Here's how the part is built. I have some questions about the finished solid (model axes, mm). Face numbers are marked on the shaded views. A direction names the side the tool comes from. Round coordinates to 2 decimals unless told otherwise and drop trailing zeros. Write each loop counter-clockwise with the first axis right and the second up, starting at its lowest first coordinate (ties: lowest second). Pieces come first, ordered by that corner, then holes. Notation, with made-up numbers: (-6.75, 20) -> (52.25, 20) arc R21 ccw to (52.25, 51) -> close; hole circle Ø5 at (44.5, 78.5). An arc over 180 degrees is marked (long way). Answer as CSV lines item,"result".
```python
from build123d import *

# Parameters (mm, degrees)
SKETCH1_R               = 3.75
SKETCH1_R_2             = 2.5
BOSS_EXTRUDE1_DEPTH     = 3
SKETCH2_R               = 5
SKETCH2_R_2             = 1.25
BOSS_EXTRUDE2_DEPTH     = 20
CUT_EXTRUDE1_START      = -19
SKETCH3_R               = 3.75
CUT_EXTRUDE1_DEPTH      = 19
CHAMFER1_SIZE           = 1.5
CUT_EXTRUDE2_DEPTH      = 25.062418831
CUT_EXTRUDE2_DEPTH_BACK = 25.062418831
SKETCH4_W               = 0.5
SKETCH4_H               = 32.118567902


with BuildPart() as part:
    # Sketch1 → Boss-Extrude1 (new body)
    with BuildSketch(Plane(origin=(0, 0, 0), x_dir=(1, 0, 0), z_dir=(0, 1, 0))):
        with Locations(Location((0, 0, 0), (0, 0, 270))):
            Circle(SKETCH1_R)
        with Locations(Location((0, 0, 0), (0, 0, 270))):
            Circle(SKETCH1_R_2, mode=Mode.SUBTRACT)
    extrude(amount=BOSS_EXTRUDE1_DEPTH)

    # Sketch2 → Boss-Extrude2 (add)
    with BuildSketch(Plane(origin=(0, 3, 0), x_dir=(1, 0, 0), z_dir=(0, 1, 0))):
        with Locations(Location((0, 0, 0), (0, 0, 270))):
            Circle(SKETCH2_R)
        with Locations(Location((0, 0, 0), (0, 0, 270))):
            Circle(SKETCH2_R_2, mode=Mode.SUBTRACT)
    extrude(amount=BOSS_EXTRUDE2_DEPTH)

    # Sketch3 → Cut-Extrude1 (cut)
    with BuildSketch(Plane(origin=(0, 23, 0), x_dir=(1, 0, 0), z_dir=(0, 1, 0)).offset(CUT_EXTRUDE1_START)):
        with Locations(Location((0, 0, 0), (0, 0, 270))):
            Circle(SKETCH3_R)
    extrude(amount=CUT_EXTRUDE1_DEPTH, mode=Mode.SUBTRACT)

    # Chamfer1
    # the kernel refuses this chamfer: 1.5 mm, written as the material it adds along each edge
    with BuildSketch(Plane(origin=(0, 3, 0), x_dir=(0, 0, 1), z_dir=(-1, 0, 0))) as chamfer1_piece_1_section:
        Polygon((3.75 + CHAMFER1_SIZE, 0), (3.75, -CHAMFER1_SIZE), (3.75, 0), align=None)
    chamfer1_piece_1 = revolve(axis=Axis((0, 3, 0), (0, 1, 0)), mode=Mode.PRIVATE)
    chamfer1_piece_1 = chamfer1_piece_1 & Plane(origin=(0, 2.126111001, 0), x_dir=(0, 0, 1), z_dir=(0, -1, 0)) * Cylinder(5, 22, mode=Mode.PRIVATE)
    add(chamfer1_piece_1)
    with BuildSketch(Plane(origin=(0, 4, 0), x_dir=(0, 0, 1), z_dir=(-1, 0, 0))) as chamfer1_piece_2:
        Polygon((3.75, CHAMFER1_SIZE), (3.75 - CHAMFER1_SIZE, 0), (3.75, 0), align=None)
    revolve(axis=Axis((0, 4, 0), (0, 1, 0)))

    # Sketch4 → Cut-Extrude2 (cut, two sides: drawn at the far end of the back side and taken through both)
    with BuildSketch(Plane.XY.offset(-CUT_EXTRUDE2_DEPTH_BACK)):
        with Locations((0, 23)):
            Rectangle(SKETCH4_W, SKETCH4_H)
    extrude(amount=CUT_EXTRUDE2_DEPTH + CUT_EXTRUDE2_DEPTH_BACK, mode=Mode.SUBTRACT)


solid = part.part
```
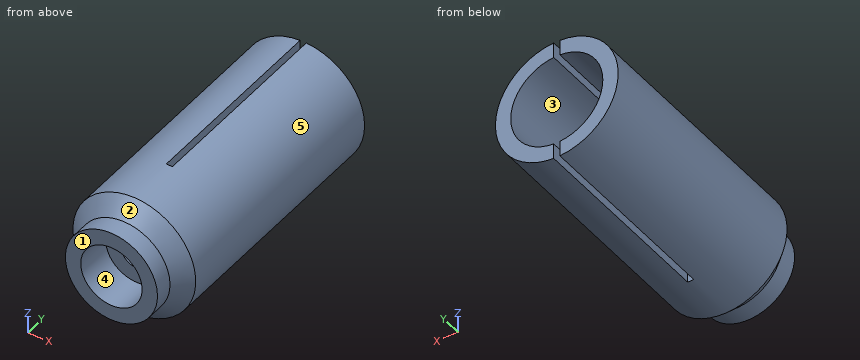
1. Suppose I cut it at B-B on z = 0. Please give me the cut outline in (x, y), and give its area (3 significant figures).
Numbers:
outline,"(-5, 2.75) -> (-3.75, 1.5) -> (-3.75, 0) -> (-2.5, 0) -> (-2.5, 3) -> (-1.25, 3) -> (-1.25, 4) -> (-2.25, 4) -> (-3.75, 5.5) -> (-3.75, 23) -> (-5, 23) -> close; (1.25, 3) -> (2.5, 3) -> (2.5, 0) -> (3.75, 0) -> (3.75, 1.5) -> (5, 2.75) -> (5, 23) -> (3.75, 23) -> (3.75, 5.5) -> (2.25, 4) -> (1.25, 4) -> close"
area,"66.9 mm^2"
2. If we mould it in two halves opening along Z, with no side actions, what happens to the marked faces 1, 2 and 3? For each: released by +Z, released by -Z, zero draft, split by the parting line, or undercut.
Numbers:
face 1,"zero draft"
face 2,"split by the parting line"
face 3,"undercut"
3. If I drill on line 1 (X direction, y = 20.75, z = 0.5); line 2 (X direction, y = 21.75, z = -4.5); line 3 (Z direction, x = 3, y = 10.5), over which ranges is the centre line in solid material (lowest first)?
Numbers:
line 1,"x = -4.97 to -3.72, 3.72 to 4.97"
line 2,"x = -2.18 to -0.25, 0.25 to 2.18"
line 3,"z = -4 to -2.25, 2.25 to 4"
4. For pin 1 Ø1.5 at (x, z) = (1, 1) entering from -Y; pin 2 Ø5 at (x, z) = (-0.5, -0.5) entering from +Y; pin 3 Ø1.5 at (y, z) = (7.5, 2) entering from -X; pin 4 Ø2 at (x, z) = (0, 0) entering from -Y (1 decimal), each with a flat end and sliding along its axis, tell me the tip position at first contact or that it passes through.
Numbers:
pin 1,"stops at y = 3"
pin 2,"stops at y = 4.96"
pin 3,"stops at x = -4.84"
pin 4,"passes through"
5. On a 3-axis mill with a long thin cutter (end or side, diameter ignored), from which of +Z, -Z, +X, -X, +Y, -Y can I reach the whole of each face in a straight line? I mean the marked faces 4 and 5. Say none if no direction works.
Numbers:
face 4,"-Y"
face 5,"+Y, -Y"
6. Suppose I cut it at C-C on x = 0. Please give me the cut outline in (y, z).
Numbers:
outline,"(0, -3.75) -> (1.5, -3.75) -> (2.75, -5) -> (6.94, -5) -> (6.94, -3.75) -> (5.5, -3.75) -> (4, -2.25) -> (4, -1.25) -> (3, -1.25) -> (3, -2.5) -> (0, -2.5) -> close; (0, 2.5) -> (3, 2.5) -> (3, 1.25) -> (4, 1.25) -> (4, 2.25) -> (5.5, 3.75) -> (6.94, 3.75) -> (6.94, 5) -> (2.75, 5) -> (1.5, 3.75) -> (0, 3.75) -> close"
